```python
from build123d import *

# Parameters (mm, degrees)
F1_DEPTH  = 25.4
F2_W      = 71.12
F2_H      = 27.3908400369
F3_DEPTH  = 50.8
F4_R      = 8.0648205789
F5_DEPTH  = 50.8
F7_DEPTH  = 50.8
F8_W      = 25.4
F8_H      = 19.05
F9_DEPTH  = 177.8
F10_W     = 12.7
F10_H     = 177.8
F11_DEPTH = 6.35
F12_W     = 6.35
F12_H     = 146.05
F13_DEPTH = 28.576
F15_DEPTH = 6.35
F17_DEPTH = 6.35


with BuildPart() as f1:
    # F0 (on Front) → F1 (new body, symmetric)
    with BuildSketch(Plane.XZ):
        Polygon((30.48, -19.05), (49.53, -19.05), (49.53, 19.05), (-49.53, 19.05), (-49.53, -19.05), (-30.48, -19.05), (-30.48, 6.35), (30.48, 6.35), align=None)
    extrude(amount=F1_DEPTH, both=True)

    # F2 (on Front) → F3 (cut, symmetric)
    with BuildSketch(Plane.XZ):
        with Locations((0, -20.0454200185)):
            Rectangle(F2_W, F2_H)
    extrude(amount=F3_DEPTH, both=True, mode=Mode.SUBTRACT)

    # F4 (on face) → F5 (join)
    with BuildSketch(Plane.XZ.offset(25.4)):
        with Locations((-35.56, -6.35)):
            Circle(F4_R)
    extrude(amount=-F5_DEPTH)

    # F6 (on face) → F7 (join)
    with BuildSketch(Plane.XZ.offset(25.4)):
        Polygon((35.56, -17.4720194191), (35.56, -6.35), (30.48, -6.35), align=None)
    extrude(amount=-F7_DEPTH)

    # F8 (on face) → F9 (join)
    with BuildSketch(Plane.XY.offset(19.05)):
        with Locations((-36.83, 0)):
            Rectangle(F8_W, F8_H)
    extrude(amount=F9_DEPTH)

    # F10 (on face) → F11 (cut)
    with BuildSketch(Plane(origin=(0, 9.525, 0), x_dir=(-1, 0, 0), z_dir=(0, 1, 0))):
        with Locations((36.83, 133.35)):
            Rectangle(F10_W, F10_H)
    extrude(amount=-F11_DEPTH, mode=Mode.SUBTRACT)

    # F12 (on face) → F13 (cut, through all)
    with BuildSketch(Plane(origin=(0, 3.175, 0), x_dir=(-1, 0, 0), z_dir=(0, 1, 0))):
        with Locations((36.83, 117.475)):
            Rectangle(F12_W, F12_H)
    extrude(amount=-F13_DEPTH, mode=Mode.SUBTRACT)

    # F14 (on face) → F15 (join)
    with BuildSketch(Plane(origin=(-49.53, 0, 0), x_dir=(0, -1, 0), z_dir=(-1, 0, 0))):
        Polygon((-25.4, 19.05), (-9.525, 19.05), (-9.525, 44.45), align=None)
        Polygon((25.4, 19.05), (9.525, 44.45), (9.525, 19.05), align=None)
    extrude(amount=-F15_DEPTH)

    # F16 (on face) → F17 (join)
    with BuildSketch(Plane.YZ.offset(-24.13)):
        Polygon((-25.3417864442, 19.05), (-9.525, 19.05), (-9.525, 44.45), align=None)
        Polygon((9.525, 43.8476071775), (9.525, 19.05), (25.4153106362, 19.05), align=None)
    extrude(amount=-F17_DEPTH)


solid = f1.part
```
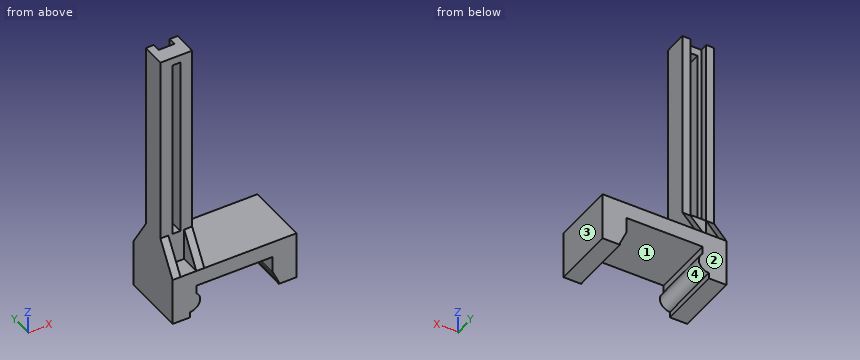
Check sheet for the modelled part. Datum: model origin and axes. Units: mm. Face numbers are marked on the shaded views. Coordinates: 2 decimals unless noted, no trailing zeros. Order: outer loops, then holes, each group sorted by start corner. A loop starts at its lowest first (then second) coordinate and runs counter-clockwise, first axis right, second up. Notation, with made-up numbers: M 84.5,85 L 100.5,85 A12 ccw 100.5,94 Z; hole C -29,7 d3. An arc over 180 degrees is marked long. Write each question's results on one line, items separated by ' | '. Start each with the question number.
1. Material ranges on probe 1 along X at (y, z) = (3, 84) (3 decimals); probe 2 along X at (y, z) = (5, 51); probe 3 along Z at (x, y) = (-35.5, -5), recorded low to high.
2. Cross-section at B-B on y = -2. Record the cut outline in (x, z) (3 decimals).
3. Cross-section at C-C on y = 14. Record the cut outline in (x, z), and give its area (3 significant figures).
4. Go/stop test with flat-tipped pins: P1, Ø1, axis at x = 38, y = -1, coming from the +Z side; P2, Ø15, axis at x = -12.5, y = -7, coming from the -Z side; P3, Ø6.5, axis at x = -39, z = 115.5, coming from the +Y side (3 decimals). Record where each tip stops, or that it passes through.
5. Cross-section at A-A on z = 61.5. Record the cut outline in (x, y) (3 decimals), and give its area (3 significant figures).
6. Mould release check, pull along X, two halves, no side actions. Record for the marked faces 1, 2, 3 and 4: +X half, -X half, draft (parallel to the pull), parting line (faces both ways), or undercut.
7. Cross-section at D-D on x = 9.5. Record the cut outline in (y, z), and give its area (3 significant figures).
Checks:
1) probe 1: x = -49.53 to -40.005, -33.655 to -24.13 | probe 2: x = -49.53 to -43.18, -30.48 to -24.13 | probe 3: z = -14.41 to 44.45, 190.5 to 196.85
2) outline: M -49.53,-19.05 L -35.56,-19.05 L -35.56,-14.415 A8.065 ccw -30.48,-0.086 L -30.48,6.35 L 30.48,6.35 L 30.48,-6.35 L 35.56,-17.472 L 35.56,-19.05 L 49.53,-19.05 L 49.53,19.05 L -24.13,19.05 L -24.13,196.85 L -49.53,196.85 Z; hole M -40.005,44.45 L -33.655,44.45 L -33.655,190.5 L -40.005,190.5 Z
3) outline: M -49.53,-19.05 L -35.56,-19.05 L -35.56,-14.41 A8.06 ccw -30.48,-0.09 L -30.48,6.35 L 30.48,6.35 L 30.48,-6.35 L 35.56,-17.47 L 35.56,-19.05 L 49.53,-19.05 L 49.53,19.05 L -24.13,19.05 L -24.13,36.86 L -30.48,36.86 L -30.48,19.05 L -43.18,19.05 L -43.18,37.29 L -49.53,37.29 Z | area: 2,420 mm²
4) P1: stops at z = 19.05 | P2: stops at z = 6.35 | P3: stops at y = 3.175
5) outline: M -49.53,-9.525 L -40.005,-9.525 L -40.005,3.175 L -43.18,3.175 L -43.18,9.525 L -49.53,9.525 Z; M -33.655,-9.525 L -24.13,-9.525 L -24.13,9.525 L -30.48,9.525 L -30.48,3.175 L -33.655,3.175 Z | area: 323 mm²
6) face 1: undercut | face 2: draft | face 3: +X half | face 4: undercut
7) outline: M -25.4,6.35 L 25.4,6.35 L 25.4,19.05 L -25.4,19.05 Z | area: 645 mm²
